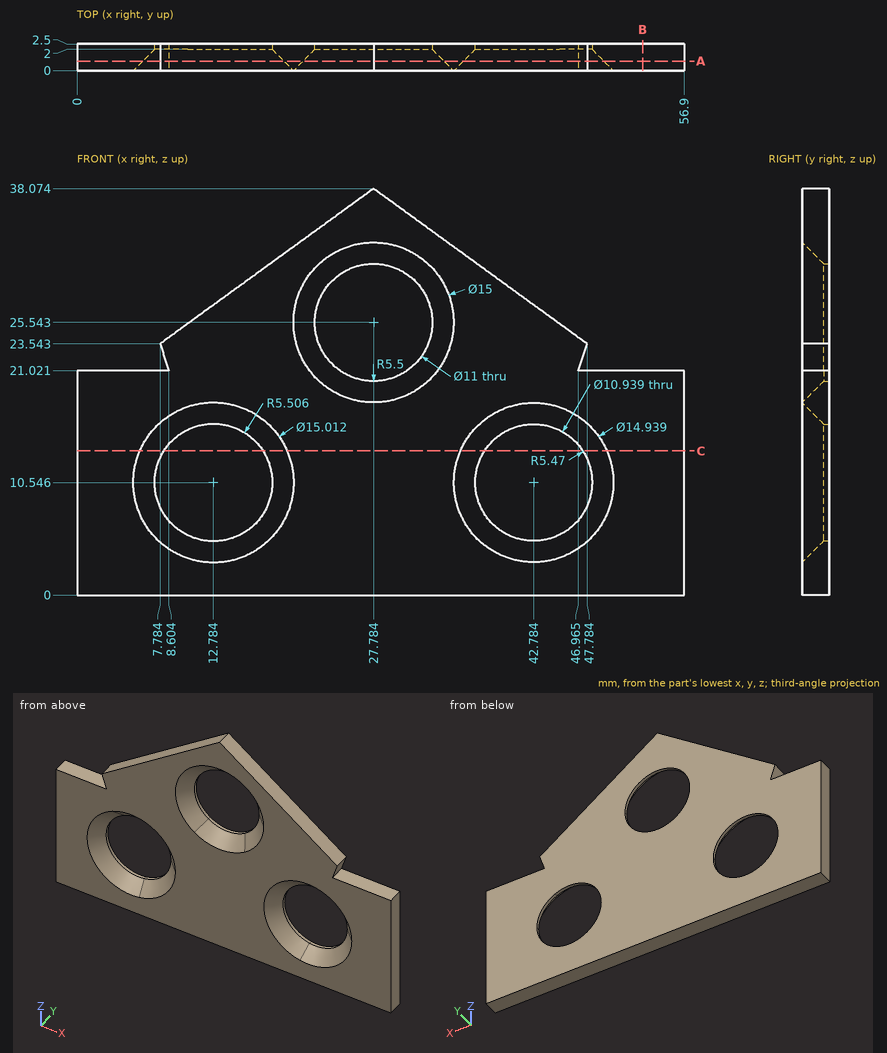
The figure shows three views and two pictorial views of one solid part (mm, origin at its lowest corner). Answer the questions. Give positions to 0.01 mm unless a question says otherwise; leave off trailing zeros. Order: outer loops, then holes, each group sorted by start corner. A loop starts at its lowest first (then second) coordinate and runs counter-clockwise, first axis right, second up. Notation, with made-up numbers: (53.25, 34.25) - (112.25, 34.25) arc R18 cw to (112.25, 52.25) - close; hole circle Ø4 at (40, 34). An arc over 180 degrees is marked (long way). Answer as CSV lines item,"result".
Q1. Straight lines are drawn through the part: L1, parallel to X at y = 1.1, z = 14 (1 decimal); L2, parallel to X at y = 0.85, z = 6.5 (1 decimal); L3, parallel to Z at x = 30, y = 0.4 (1 decimal). For each, find the intervals that lie inside material, in ascending order.
Answer key:
L1,"x = 0 to 7.4, 18.2 to 37.4, 48.1 to 56.9"
L2,"x = 0 to 7.5, 18.1 to 37.5, 48 to 56.9"
L3,"z = 0 to 18.8, 32.3 to 36.5"
Q2. A cutting plane is placed at B-B, the plane x = 53. Determine the outline of the cut face in (y, z).
Answer key:
outline,"(0, 0) - (2.5, 0) - (2.5, 21.02) - (0, 21.02) - close"
Q3. Each of these flat-tipped pins is pushed along its axis until it touches: pin 1 Ø0.8 at (x, y) = (51, 1) entering from +Z; pin 2 Ø1.5 at (x, y) = (11, 1.5) entering from +Z (1 decimal); pin 3 Ø12 at (x, z) = (17, 12) entering from -Y; pin 4 Ø9 at (x, z) = (42.78, 10.55) entering from +Y. Where does it stop, or does it pass through?
Answer key:
pin 1,"stops at z = 21.02"
pin 2,"stops at z = 26.4"
pin 3,"stops at y = 0"
pin 4,"passes through"
Q4. A cutting plane is placed at C-C, the plane z = 13.5. Count the separate pieces of the cut face and the enclosed holes in it.
Answer key:
separate pieces,"3"
enclosed holes,"0"
Q5. A cutting plane is placed at A-A, the plane y = 0.9. Determine the outline of the cut face in (x, z) (1 decimal).
Answer key:
outline,"(0, 0) - (56.9, 0) - (56.9, 21) - (47, 21) - (47.8, 23.5) - (27.8, 38.1) - (7.8, 23.5) - (8.6, 21) - (0, 21) - close; hole circle Ø13.2 at (12.8, 10.5); hole circle Ø13.2 at (27.8, 25.5); hole circle Ø13.1 at (42.8, 10.5)"
